Design review of the part built by this model. Coordinates are the model's own, in mm. Face numbers are marked on the shaded views. A direction names the side the tool comes from. Coordinates: 2 decimals unless noted, no trailing zeros. Write each loop counter-clockwise with the first axis right and the second up, starting at its lowest first coordinate (ties: lowest second). Pieces come first, ordered by that corner, then holes. Notation, with made-up numbers: (89.5, -0.5) - (142.5, -0.5) arc R25 cw to (142.5, 15.5) - close; hole circle Ø1 at (38, 13.5). An arc over 180 degrees is marked (long way). One line per item, written item: value.
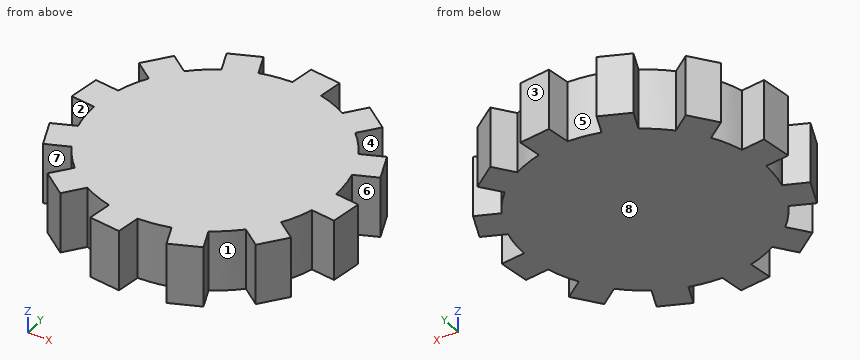
from build123d import *

# Parameters (mm, degrees)
F1_DEPTH = 3.175
F2_COUNT = 12


# Not quite as in the source:
# - a length typed as a fraction of an inch, garbled in the dataset ("3 / 203.2 mm" for 3/8 in), is restored


with BuildPart() as f1:
    # F0 (on Top) → F1 (new body)
    with BuildSketch(Plane.XY):
        with BuildLine():
            ThreePointArc((0, 6.35), (-4.4901280605, -4.4901280605), (6.35, 0))
            ThreePointArc((6.35, 0), (5.0377937108, 3.8656350742), (1.6435009364, 6.1336289969))
            ThreePointArc((1.6435009364, 6.1336289969), (0.8288413206, 6.2956748697), (0, 6.35))
        make_face()
        with BuildLine():
            ThreePointArc((0, 6.35), (0.8288413206, 6.2956748697), (1.6435009364, 6.1336289969))
            Line((1.6435009364, 6.1336289969), (1.8104587787, 7.4017997143))
            Line((1.8104587787, 7.4017997143), (0.1669578423, 7.6181707174))
            Line((0.1669578423, 7.6181707174), (0, 6.35))
        make_face()
    extrude(amount=F1_DEPTH)

    # F2: F1 ×12 about axis
    f2_axis = Axis((0, 0, 0), (0, 0, -1))


with BuildPart() as f1_1:
    add(f1.part)
    for i in range(1, F2_COUNT):
        add(f1.part.rotate(f2_axis, i * 360 / F2_COUNT))


solid = f1_1.part
1. Consider section D-D, the plane x = 0.5. Write out the cut boundary in (y, z) (3 decimals), then the cut area to 3 significant figures.
Answer block:
outline: (-6.33, 0) - (7.574, 0) - (7.574, 3.175) - (-6.33, 3.175) - close
area: 44.1 mm^2
2. Consider section A-A, the plane x = 5. Write out the cut boundary in (y, z) (3 decimals), then the cut area to 3 significant figures.
Answer block:
outline: (-4.881, 0) - (3.914, 0) - (3.914, 3.175) - (-4.881, 3.175) - close; (5.155, 0) - (5.711, 0) - (5.711, 3.175) - (5.155, 3.175) - close
area: 29.7 mm^2
3. Mouldability with a two-part tool opening along Y and no side actions: class the marked faces 6, 7 and 8 as released by +Y, released by -Y, zero draft, split by the parting line, or undercut.
Answer block:
face 6: undercut
face 7: released by -Y
face 8: zero draft
4. Consider section B-B, the plane y = 0.5. Write out the cut boundary in (x, z) (3 decimals).
Answer block:
outline: (-7.574, 0) - (6.33, 0) - (6.33, 3.175) - (-7.574, 3.175) - close
5. For the marked faces 1, 2, 3, 4 and 5, list the 3-axis set-ups (+Z, -Z, +X, -X, +Y, -Y) from which the entire face can be reached by the end or side of a thin tool; tool diameter is ignored.
Answer block:
face 1: +Z, -Z
face 2: +Z, -Z, -X
face 3: +Z, -Z, +X, +Y
face 4: +Z, -Z, +X
face 5: +Z, -Z, +Y
6. Wall thickness on line 1 along X through (y, z) = (3.25, 2.8); line 2 along X through (y, z) = (5.75, 2.55); line 3 along Y through (x, z) = (4.75, 0.7): over which ranges is each line inside the solid? List them lowest first.
Answer block:
line 1: x = -5.6 to 5.46, 5.68 to 6.85
line 2: x = -3.28 to 2.69, 3.37 to 4.95
line 3: y = -4.69 to 4.21, 4.83 to 5.9
7. Consider section C-C, the plane x = -4.75. Write out the cut boundary in (y, z) (3 decimals), then the cut area to 3 significant figures.
Answer block:
outline: (-5.903, 0) - (-4.829, 0) - (-4.829, 3.175) - (-5.903, 3.175) - close; (-4.214, 0) - (4.69, 0) - (4.69, 3.175) - (-4.214, 3.175) - close
area: 31.7 mm^2
